```python
from build123d import *

# Parameters (mm, degrees)
F1_W     = 5
F1_H     = 10
F1_R     = 1.6
F1_W_2   = 10
F1_H_2   = 5
F2_DEPTH = 5


with BuildPart() as f2:
    # F1 (on Front) → F2 (new body)
    with BuildSketch(Plane.XZ):
        with BuildLine():
            Line((-21, 35), (-21, 27))
            ThreePointArc((-21, 27), (-22.4644660941, 23.4644660941), (-26, 22))
            Line((-26, 22), (-26, 2))
            Line((-26, 2), (-46, 2))
            Line((-46, 2), (-46, 22))
            Line((-46, 22), (-51, 22))
            Line((-51, 22), (-51, -5))
            ThreePointArc((-51, -5), (-50.1213203436, -7.1213203436), (-48, -8))
            Line((-48, -8), (38, -8))
            ThreePointArc((38, -8), (40.1213203436, -7.1213203436), (41, -5))
            Line((41, -5), (41, 35))
            ThreePointArc((41, 35), (40.1213203436, 37.1213203436), (38, 38))
            Line((38, 38), (-18, 38))
            ThreePointArc((-18, 38), (-20.1213203436, 37.1213203436), (-21, 35))
        make_face()
        with Locations((-15.5, 0)):
            Rectangle(F1_W, F1_H, mode=Mode.SUBTRACT)
        with Locations((35.5, 0)):
            Rectangle(F1_W, F1_H, mode=Mode.SUBTRACT)
        with Locations((2.5, 10)):
            Circle(F1_R, mode=Mode.SUBTRACT)
        with Locations((17.5, 10)):
            Circle(F1_R, mode=Mode.SUBTRACT)
        with Locations((-15.5, 15)):
            Circle(F1_R, mode=Mode.SUBTRACT)
        with Locations((-15.5, 30)):
            Rectangle(F1_W, F1_H, mode=Mode.SUBTRACT)
        with Locations((2.5, 20)):
            Circle(F1_R, mode=Mode.SUBTRACT)
        with Locations((10, 15)):
            Rectangle(F1_W_2, F1_H_2, mode=Mode.SUBTRACT)
        with Locations((17.5, 20)):
            Circle(F1_R, mode=Mode.SUBTRACT)
        with Locations((35.5, 15)):
            Circle(F1_R, mode=Mode.SUBTRACT)
        with Locations((35.5, 30)):
            Rectangle(F1_W, F1_H, mode=Mode.SUBTRACT)
    extrude(amount=F2_DEPTH)


solid = f2.part
```
Check sheet for the modelled part. Datum: model origin and axes. Units: mm. A direction names the side the tool comes from. Round coordinates to 2 decimals unless told otherwise and drop trailing zeros. Loops run counter-clockwise (first coordinate to the right, second up) from the corner with the lowest first, then second, coordinate; pieces in that order, holes last. Notation, with made-up numbers: (-1.5, 47) - (34.5, 47) arc R20 ccw to (34.5, 82) - close; hole circle Ø8 at (-1.75, 0.25). An arc over 180 degrees is marked (long way). Write item = value, one per line. Start each with the question number.
Q1. Release check for a two-part mould opening along X. For faces 4 (the face through (-21, -2, 31)), 5 (the face through (5, -2, 15)), 6 (the face through (-48, -2, 22)) record: pulls with the +X half, pulls with the -X half, needs draft (parallel to the pull), parting line crosses it, or undercut.
Q2. Section check A-A (x = 6). Record the boundary of the cut face in (y, z), plus the area to 3 significant figures.
Q3. Access from +Z, -Z, +X, -X, +Y, -Y to the whole of each face (thin tool, end or side, straight path). Record for faces 1 (the face through (-36, -2, 2)), 2 (the face through (10, -2, 12.5)), 3 (the face through (-20.1, -2.46, 37.14)).
Q4. Section check D-D (z = 15). Record the boundary of the cut face in (x, y).
Q5. Section check C-C (x = 17.5). Record the boundary of the cut face in (y, z).
Q6. Thickness scan on L1, parallel to X at y = -1.85, z = 32.5; L2, parallel to Z at x = 17.5, y = -2; L3, parallel to X at y = -2.6, z = 17. Record the ranges inside material, lowest first.
Q7. Depth check by flat-ended pin: P1, Ø1.5, axis at y = -2, z = 28.5, coming from the -X side; P2, Ø5, axis at x = 5.5, z = 19, coming from the +Y side; P3, Ø2.5, axis at x = -49.5, y = -3.5, coming from the +Z side; P4, Ø3, axis at x = 17.5, z = 10, coming from the +Y side. Enter the tip coordinate at first touch or a pass-through.
Q8. Section check B-B (z = 10). Record the boundary of the cut face in (x, y).
Derived:
q1.face_4 = pulls with the -X half
q1.face_5 = undercut
q1.face_6 = needs draft
q2.outline = (-5, -8) - (0, -8) - (0, 12.5) - (-5, 12.5) - close; (-5, 17.5) - (0, 17.5) - (0, 38) - (-5, 38) - close
q2.area = 205 mm^2
q3.face_1 = +Z, +Y, -Y
q3.face_2 = +Y, -Y
q3.face_3 = +Z, -X, +Y, -Y
q4.outline = (-51, -5) - (-46, -5) - (-46, 0) - (-51, 0) - close; (-26, -5) - (-17.1, -5) - (-17.1, 0) - (-26, 0) - close; (-13.9, -5) - (5, -5) - (5, 0) - (-13.9, 0) - close; (15, -5) - (33.9, -5) - (33.9, 0) - (15, 0) - close; (37.1, -5) - (41, -5) - (41, 0) - (37.1, 0) - close
q5.outline = (-5, -8) - (0, -8) - (0, 8.4) - (-5, 8.4) - close; (-5, 11.6) - (0, 11.6) - (0, 18.4) - (-5, 18.4) - close; (-5, 21.6) - (0, 21.6) - (0, 38) - (-5, 38) - close
q6.L1 = -21 to -18, -13 to 33, 38 to 41
q6.L2 = -8 to 8.4, 11.6 to 18.4, 21.6 to 38
q6.L3 = -51 to -46, -26 to 5, 15 to 41
q7.P1 = -21
q7.P2 = 0
q7.P3 = 22
q7.P4 = through
q8.outline = (-51, -5) - (-46, -5) - (-46, 0) - (-51, 0) - close; (-26, -5) - (0.9, -5) - (0.9, 0) - (-26, 0) - close; (4.1, -5) - (15.9, -5) - (15.9, 0) - (4.1, 0) - close; (19.1, -5) - (41, -5) - (41, 0) - (19.1, 0) - close
